from build123d import *

# Parameters (mm, degrees)
F1_R     = 17.315
F2_DEPTH = 0.8
F3_DEPTH = 15
F4_DEPTH = 12
F5_SIZE  = 0.48
F6_SIZE  = 0.48


with BuildPart() as f2:
    # F1 (on Top) → F2 (new body)
    with BuildSketch(Plane.XY):
        Circle(F1_R)
        with BuildLine():
            ThreePointArc((16.3501077978, 0.4), (16.3537769037, 0.200014958), (16.355, 0))
            ThreePointArc((16.355, 0), (16.3537769037, -0.200014958), (16.3501077978, -0.4))
            ThreePointArc((16.3501077978, -0.4), (11.5647314063, -11.5647314063), (0.4, -16.3501077978))
            ThreePointArc((0.4, -16.3501077978), (0, -16.355), (-0.4, -16.3501077978))
            ThreePointArc((-0.4, -16.3501077978), (-11.5647314063, -11.5647314063), (-16.3501077978, -0.4))
            ThreePointArc((-16.3501077978, -0.4), (-16.355, 0), (-16.3501077978, 0.4))
            ThreePointArc((-16.3501077978, 0.4), (-11.5647314063, 11.5647314063), (-0.4, 16.3501077978))
            ThreePointArc((-0.4, 16.3501077978), (0, 16.355), (0.4, 16.3501077978))
            ThreePointArc((0.4, 16.3501077978), (11.5647314063, 11.5647314063), (16.3501077978, 0.4))
        make_face(mode=Mode.SUBTRACT)
        with BuildLine():
            Line((15.8699598298, 0.4), (16.3501077978, 0.4))
            ThreePointArc((16.3501077978, 0.4), (11.5647314063, 11.5647314063), (0.4, 16.3501077978))
            Line((0.4, 16.3501077978), (0.4, 15.8699598298))
            Line((0.4, 15.8699598298), (-0.4, 15.8699598298))
            Line((-0.4, 15.8699598298), (-0.4, 16.3501077978))
            ThreePointArc((-0.4, 16.3501077978), (-11.5647314063, 11.5647314063), (-16.3501077978, 0.4))
            Line((-16.3501077978, 0.4), (-15.8699598298, 0.4))
            Line((-15.8699598298, 0.4), (-15.8699598298, -0.4))
            Line((-15.8699598298, -0.4), (-16.3501077978, -0.4))
            ThreePointArc((-16.3501077978, -0.4), (-11.5647314063, -11.5647314063), (-0.4, -16.3501077978))
            Line((-0.4, -16.3501077978), (-0.4, -15.8699598298))
            Line((-0.4, -15.8699598298), (0.4, -15.8699598298))
            Line((0.4, -15.8699598298), (0.4, -16.3501077978))
            ThreePointArc((0.4, -16.3501077978), (11.5647314063, -11.5647314063), (16.3501077978, -0.4))
            Line((16.3501077978, -0.4), (15.8699598298, -0.4))
            Line((15.8699598298, -0.4), (15.8699598298, 0.4))
        make_face()
        with BuildLine():
            Line((-15.8699598298, 0.4), (-16.3501077978, 0.4))
            ThreePointArc((-16.3501077978, 0.4), (-16.355, 0), (-16.3501077978, -0.4))
            Line((-16.3501077978, -0.4), (-15.8699598298, -0.4))
            Line((-15.8699598298, -0.4), (-15.8699598298, 0.4))
        make_face()
        with BuildLine():
            ThreePointArc((-0.4, -16.3501077978), (0, -16.355), (0.4, -16.3501077978))
            Line((0.4, -16.3501077978), (0.4, -15.8699598298))
            Line((0.4, -15.8699598298), (-0.4, -15.8699598298))
            Line((-0.4, -15.8699598298), (-0.4, -16.3501077978))
        make_face()
        with BuildLine():
            ThreePointArc((16.3501077978, -0.4), (16.3537769037, -0.200014958), (16.355, 0))
            ThreePointArc((16.355, 0), (16.3537769037, 0.200014958), (16.3501077978, 0.4))
            Line((16.3501077978, 0.4), (15.8699598298, 0.4))
            Line((15.8699598298, 0.4), (15.8699598298, -0.4))
            Line((15.8699598298, -0.4), (16.3501077978, -0.4))
        make_face()
        with BuildLine():
            Line((0.4, 15.8699598298), (0.4, 16.3501077978))
            ThreePointArc((0.4, 16.3501077978), (0, 16.355), (-0.4, 16.3501077978))
            Line((-0.4, 16.3501077978), (-0.4, 15.8699598298))
            Line((-0.4, 15.8699598298), (0.4, 15.8699598298))
        make_face()
    extrude(amount=-F2_DEPTH)

    # F1 (on Top) → F3 (join)
    with BuildSketch(Plane.XY):
        Circle(F1_R)
        with BuildLine():
            ThreePointArc((16.3501077978, 0.4), (16.3537769037, 0.200014958), (16.355, 0))
            ThreePointArc((16.355, 0), (16.3537769037, -0.200014958), (16.3501077978, -0.4))
            ThreePointArc((16.3501077978, -0.4), (11.5647314063, -11.5647314063), (0.4, -16.3501077978))
            ThreePointArc((0.4, -16.3501077978), (0, -16.355), (-0.4, -16.3501077978))
            ThreePointArc((-0.4, -16.3501077978), (-11.5647314063, -11.5647314063), (-16.3501077978, -0.4))
            ThreePointArc((-16.3501077978, -0.4), (-16.355, 0), (-16.3501077978, 0.4))
            ThreePointArc((-16.3501077978, 0.4), (-11.5647314063, 11.5647314063), (-0.4, 16.3501077978))
            ThreePointArc((-0.4, 16.3501077978), (0, 16.355), (0.4, 16.3501077978))
            ThreePointArc((0.4, 16.3501077978), (11.5647314063, 11.5647314063), (16.3501077978, 0.4))
        make_face(mode=Mode.SUBTRACT)
    extrude(amount=F3_DEPTH)

    # F1 (on Top) → F4 (join)
    with BuildSketch(Plane.XY):
        with BuildLine():
            Line((0.4, 15.8699598298), (0.4, 16.3501077978))
            ThreePointArc((0.4, 16.3501077978), (0, 16.355), (-0.4, 16.3501077978))
            Line((-0.4, 16.3501077978), (-0.4, 15.8699598298))
            Line((-0.4, 15.8699598298), (0.4, 15.8699598298))
        make_face()
        with BuildLine():
            Line((-15.8699598298, 0.4), (-16.3501077978, 0.4))
            ThreePointArc((-16.3501077978, 0.4), (-16.355, 0), (-16.3501077978, -0.4))
            Line((-16.3501077978, -0.4), (-15.8699598298, -0.4))
            Line((-15.8699598298, -0.4), (-15.8699598298, 0.4))
        make_face()
        with BuildLine():
            ThreePointArc((16.3501077978, -0.4), (16.3537769037, -0.200014958), (16.355, 0))
            ThreePointArc((16.355, 0), (16.3537769037, 0.200014958), (16.3501077978, 0.4))
            Line((16.3501077978, 0.4), (15.8699598298, 0.4))
            Line((15.8699598298, 0.4), (15.8699598298, -0.4))
            Line((15.8699598298, -0.4), (16.3501077978, -0.4))
        make_face()
        with BuildLine():
            ThreePointArc((-0.4, -16.3501077978), (0, -16.355), (0.4, -16.3501077978))
            Line((0.4, -16.3501077978), (0.4, -15.8699598298))
            Line((0.4, -15.8699598298), (-0.4, -15.8699598298))
            Line((-0.4, -15.8699598298), (-0.4, -16.3501077978))
        make_face()
    extrude(amount=F4_DEPTH)

    # F5
    f5_edges = [f2.edges().sort_by_distance(p)[0] for p in [
        (-17.315, 0, -0.8),
    ]]
    chamfer(f5_edges, length=F5_SIZE)

    # F6
    f6_edges = [f2.edges().sort_by_distance(p)[0] for p in [
        (-15.86996, 0, 12),
        (0, 15.86996, 12),
        (15.86996, 0, 12),
        (0, -15.86996, 12),
    ]]
    chamfer(f6_edges, length=F6_SIZE)


solid = f2.part
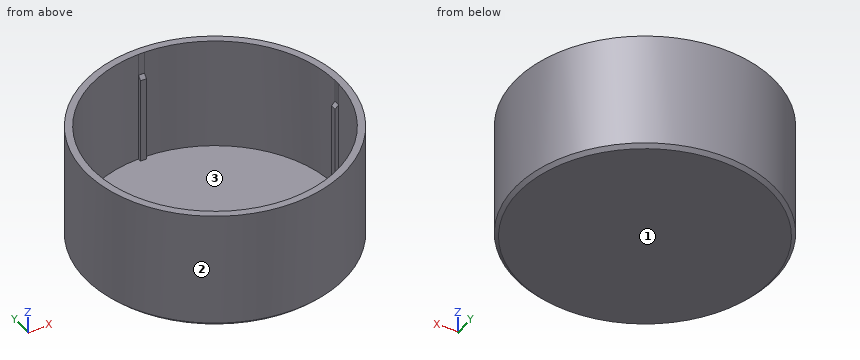
Source: CAD feature listing. Evaluate the final solid. Frame: model axes, mm. Face numbers are marked on the shaded views. Give positions to 0.01 mm unless a question says otherwise; leave off trailing zeros. Order: outer loops, then holes, each group sorted by start corner. A loop starts at its lowest first (then second) coordinate and runs counter-clockwise, first axis right, second up. Notation, with made-up numbers: (-29, 41.5) -> (-12, 41.5) arc R6 ccw to (-12, 45.5) -> close; hole circle Ø2 at (55, 52.25). An arc over 180 degrees is marked (long way). Use a Markdown table: item, result.
1) Section query A-A, the plane z = 9.5. Return the cut outline in (x, y) (3 decimals), then the cut area to 3 significant figures.
Answer list:
| item | result |
|---|---|
| outline | circle Ø34.63 at (0, 0); hole (-16.35, -0.4) arc R16.355 ccw to (-0.4, -16.35) -> (-0.4, -15.87) -> (0.4, -15.87) -> (0.4, -16.35) arc R16.355 ccw to (16.35, -0.4) -> (15.87, -0.4) -> (15.87, 0.4) -> (16.35, 0.4) arc R16.355 ccw to (0.4, 16.35) -> (0.4, 15.87) -> (-0.4, 15.87) -> (-0.4, 16.35) arc R16.355 ccw to (-16.35, 0.4) -> (-15.87, 0.4) -> (-15.87, -0.4) -> close |
| area | 103 mm² |
2) Contact query for flat-ended pins moving along their axis: P1, Ø10, axis at x = -2, y = 6.5, coming from the +Z side; P2, Ø2, axis at x = -13.5, z = 9.5, coming from the -Y side; P3, Ø0.5, axis at y = -16, z = 4.5, coming from the +X side. Output: stop coordinate, or through.
Answer list:
| item | result |
|---|---|
| P1 | z = 0 |
| P2 | y = -11.98 |
| P3 | x = 7.19 |
3) Mould query, pull axis X, two halves, no side actions, for the marked faces 1, 2 and 3. Classes: +X half, -X half, draft (parallel to the pull), parting line (faces both ways), or undercut.
Answer list:
| item | result |
|---|---|
| face 1 | draft |
| face 2 | parting line |
| face 3 | undercut |
4) Section query B-B, the plane z = 13.5. Return the cut outline in (x, y) (3 decimals), then the cut area to 3 significant figures.
Answer list:
| item | result |
|---|---|
| outline | circle Ø34.63 at (0, 0); hole circle Ø32.71 at (0, 0) |
| area | 102 mm² |
5) Ray query, line 1 along X through (y, z) = (-0.5, 2.25); line 2 along Y through (x, z) = (0, 4.5) (3 decimals); line 3 along Z through (x, y) = (8, -6). Return the intervals inside material, ascending. Write a range as [from, to].
Answer list:
| item | result |
|---|---|
| line 1 | [-17.31, -16.35], [16.35, 17.31] |
| line 2 | [-17.315, -15.87], [15.87, 17.315] |
| line 3 | [-0.8, 0] |
